Job drawing, mm, ordinate dimensions from the low corner. One solid piece. Round coordinates to 2 decimals unless told otherwise and drop trailing zeros. Order: outer loops, then holes, each group sorted by start corner. A loop starts at its lowest first (then second) coordinate and runs counter-clockwise, first axis right, second up. Notation, with made-up numbers: (22, -19) -> (34, -19) arc R29 cw to (34, 8) -> close; hole circle Ø8 at (37, 32.25). An arc over 180 degrees is marked (long way). Return JSON: item names as keys, results as strings. Group by question number.
Q1. Cut at B-B (x = 2.5). Write the cut outline in (y, z), then the cut area to 3 significant figures.
Q2. Cut at A-A (z = 2.5). Write the cut outline in (x, y), then the cut area to 3 significant figures.
Q3. Probe line 1 along X through (y, z) = (13, 2.5); line 2 along X through (y, z) = (5, 4). List the from-to ranges inside material, lowest first.
Q4. Flat gauge pin, fed straight in: pin 1 (1.5 mm diameter, centred on x = 1.5, z = 4, fed in from -Y). Where does the tip first touch, or does it go through?
Q5. Mould opens along Z. For the marked faces 1 and 2 say: +Z half, -Z half, draft (parallel to the pull), parting line (faces both ways), or undercut.
Q6. Cut at C-C (y = 8). Write the cut outline in (x, z), then the cut area to 3 significant figures.
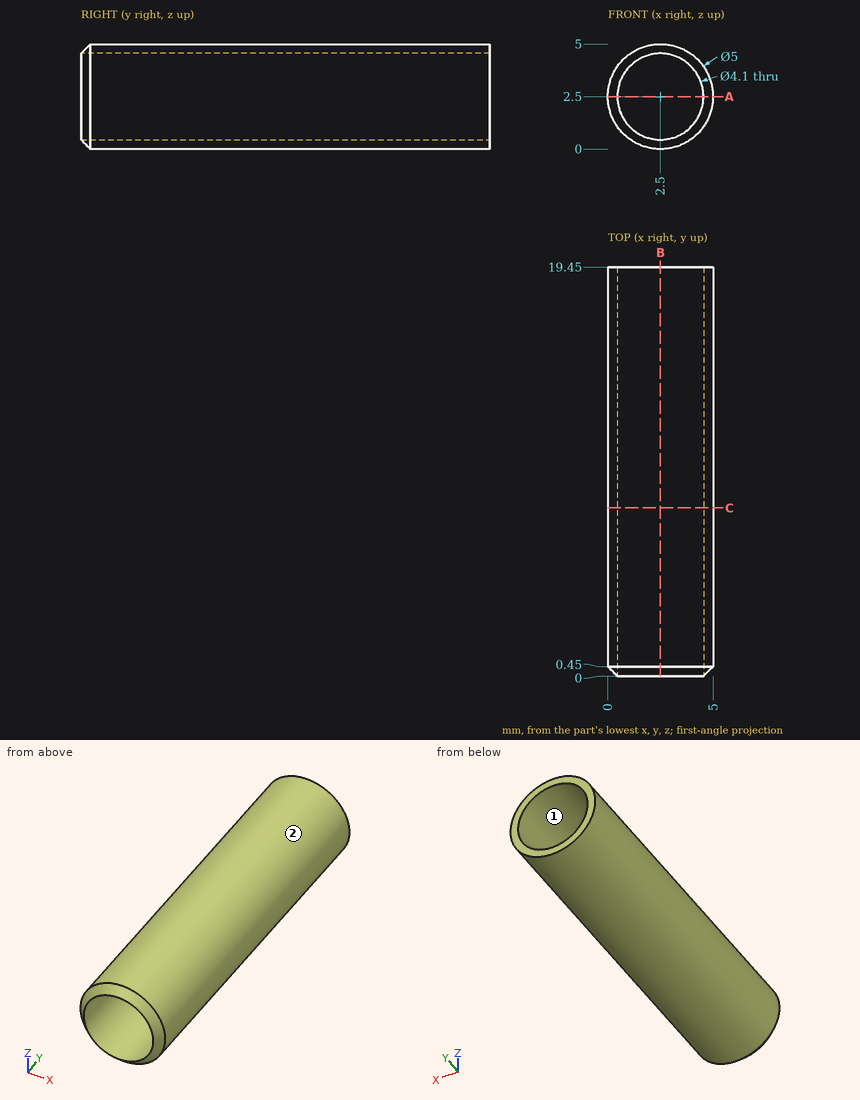
Solution:
{
 "1": {"outline": "(0, 0.45) -> (0.45, 0) -> (19.45, 0) -> (19.45, 0.45) -> close; (0, 4.55) -> (19.45, 4.55) -> (19.45, 5) -> (0.45, 5) -> close", "area": "17.3 mm²"},
 "2": {"outline": "(0, 0.45) -> (0.45, 0) -> (0.45, 19.45) -> (0, 19.45) -> close; (4.55, 0) -> (5, 0.45) -> (5, 19.45) -> (4.55, 19.45) -> close", "area": "17.3 mm²"},
 "3": {"line 1": "x = 0 to 0.45, 4.55 to 5", "line 2": "x = 0.5 to 1.1, 3.9 to 4.5"},
 "4": {"pin 1": "stops at y = 0"},
 "5": {"face 1": "undercut", "face 2": "parting line"},
 "6": {"outline": "circle Ø5 at (2.5, 2.5); hole circle Ø4.1 at (2.5, 2.5)", "area": "6.43 mm²"}
}
